Read the model definition and answer for the solid it produces. Units are mm, in the model's axes. Face numbers are marked on the shaded views. A direction names the side the tool comes from. Give positions to 0.01 mm unless a question says otherwise; leave off trailing zeros. Order: outer loops, then holes, each group sorted by start corner. A loop starts at its lowest first (then second) coordinate and runs counter-clockwise, first axis right, second up. Notation, with made-up numbers: M 37,-3.75 L 51,-3.75 A25 ccw 51,10.25 Z; hole C -14.75,59.25 d6. An arc over 180 degrees is marked long. One line per item, written item: value. Start each with the question number.
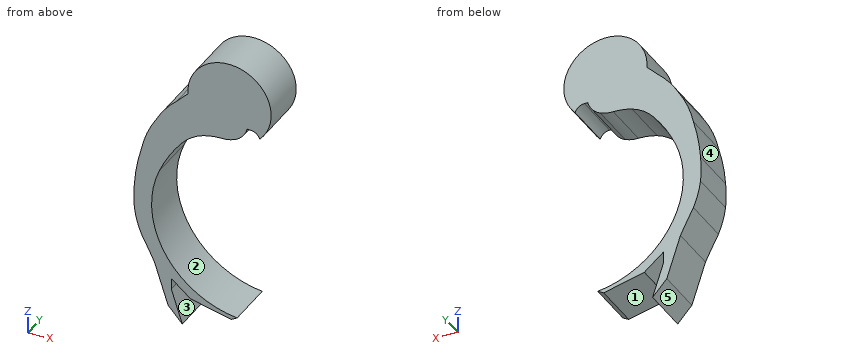
from build123d import *

# Parameters (mm, degrees)
BOSS_EXTRUDE1_DEPTH = 10


with BuildPart() as part:
    # sungu kiri → Boss-Extrude1 (new body)
    with BuildSketch(Plane(origin=(0, 0, 0), x_dir=(1, 0, 0), z_dir=(0, 1, 0))):
        with BuildLine():
            Line((-20.214241335, 18.58200887), (-17.903708636, 25.676772527))
            Line((-17.903708636, 25.676772527), (-20.879327355, 22.419581076))
            Line((-20.879327355, 22.419581076), (-23.726014444, 13.678492013))
            ThreePointArc((-23.726014444, 13.678492013), (-25.061399851, 10.98195956), (-26.444409257, 8.309539974))
            ThreePointArc((-26.444409257, 8.309539974), (-27.383764934, 5.63006722), (-27.936945566, 2.845115782))
            ThreePointArc((-27.936945566, 2.845115782), (-28.068014235, 0.18049064), (-27.936945566, -2.484134502))
            ThreePointArc((-27.936945566, -2.484134502), (-27.425713247, -6.715299694), (-26.444409257, -10.862727794))
            ThreePointArc((-26.444409257, -10.862727794), (-25.296755437, -14.61403578), (-23.488374839, -18.095297119))
            ThreePointArc((-23.488374839, -18.095297119), (-21.509226875, -21.111515913), (-19.028108575, -23.730419207))
            ThreePointArc((-19.028108575, -23.730419207), (-17.889571337, -24.893820319), (-16.718896344, -26.024877014))
            ThreePointArc((-16.718896344, -26.024877014), (-5.074889233, -34.816772241), (-1.682577981, -20.626192702))
            ThreePointArc((-1.682577981, -20.626192702), (-2.440511975, -21.639521262), (-3.645798168, -22.024987085))
            Line((-3.645798168, -22.024987085), (-4.330199558, -22.024987085))
            ThreePointArc((-4.330199558, -22.024987085), (-5.29733591, -20.16091762), (-6.958490383, -18.876132224))
            ThreePointArc((-6.958490383, -18.876132224), (-8.290108773, -18.468617913), (-9.67568618, -18.329152159))
            ThreePointArc((-9.67568618, -18.329152159), (-11.660303974, -18.169286257), (-13.595617391, -17.701496911))
            ThreePointArc((-13.595617391, -17.701496911), (-16.012005666, -16.475638304), (-18.010368345, -14.645827324))
            ThreePointArc((-18.010368345, -14.645827324), (-20.650416196, -11.005311906), (-22.72256926, -7.01414831))
            ThreePointArc((-22.72256926, -7.01414831), (-21.584958488, 10.98418111), (-6.423603233, 20.74980075))
            Line((-6.423603233, 20.74980075), (-7.667855794, 21.470443038))
            Line((-7.667855794, 21.470443038), (-16.17291449, 19.521519125))
            Line((-16.17291449, 19.521519125), (-20.214241335, 16.223172594))
            Line((-20.214241335, 16.223172594), (-20.214241335, 18.58200887))
        make_face()
    extrude(amount=BOSS_EXTRUDE1_DEPTH)


solid = part.part
Q1. A tool of negligible diameter and unlimited length cuts with its end or side. For the marked faces 1 and 2, from which of +Z, -Z, +X, -X, +Y, -Y can it reach the whole face along a straight path? Write none if from no direction.
Q2. Find section A-A, the plane y = 2.25. Give the vertices of the cut face in (x, z).
Q3. Each of these flat-tipped pins is pushed along its axis until it touches: pin 1 (3 mm diameter, centred on y = 2, z = 20, fed in from -X); pin 2 (0.7 mm diameter, centred on y = 3, z = -18, fed in from +X); pin 3 (5 mm diameter, centred on y = 9, z = -16.5, fed in from +X); pin 4 (10 mm diameter, centred on x = -12, z = -19.5, fed in from -Y). Where does it stop, or does it pass through?
Q4. Consider probe 1 along Z at (x, y) = (-9.75, 9.5); probe 2 along Z at (x, y) = (-14.75, 6.5); probe 3 along X at (y, z) = (5.75, -0.5). Determine where each line is inside the solid, lowest interval first.
Q5. Find section B-B, the plane x = -25.25. Give the vertices of the cut face in (y, z), then the cut area to 3 significant figures.
Q6. Determine the mould class of the marked faces 3, 4 and 5 for opening direction Z: released by +Z, released by -Z, zero draft, split by the parting line, or undercut.
Q7. Find section C-C, the plane z = 15.5. Give the vertices of the cut face in (x, y), then the cut area to 3 significant figures.
Evaluation:
1. face 1: -Z, +Y, -Y
1. face 2: +X, +Y, -Y
2. outline: M -27.94,-2.85 A20.14 ccw -26.44,-8.31 A169.62 cw -23.73,-13.68 L -20.88,-22.42 L -17.9,-25.68 L -20.21,-18.58 L -20.21,-16.22 L -16.17,-19.52 L -7.67,-21.47 L -6.42,-20.75 A20 cw -22.72,7.01 A30.3 cw -18.01,14.65 A10 cw -13.6,17.7 A12.71 cw -9.68,18.33 A7.09 ccw -6.96,18.88 A4.88 ccw -4.33,22.02 L -3.65,22.02 A2.08 cw -1.68,20.63 A8.72 ccw long -16.72,26.02 A58.11 ccw -19.03,23.73 A20.33 ccw -23.49,18.1 A21.56 ccw -26.44,10.86 A38.04 ccw -27.94,2.48 A27.15 ccw Z
3. pin 1: x = -23.27
3. pin 2: x = -14.04
3. pin 3: x = -12.76
3. pin 4: y = 0
4. probe 1: -20.99 to -20.11, 18.33 to 35.16
4. probe 2: -19.85 to -17.93, 17.22 to 32.15
4. probe 3: -28.07 to -24.33
5. outline: M 0,-10.61 L 10,-10.61 L 10,14.73 L 0,14.73 Z
5. area: 253 mm2
6. face 3: undercut
6. face 4: released by +Z
6. face 5: released by -Z
7. outline: M -24.91,0 L -17.21,0 L -17.21,10 L -24.91,10 Z
7. area: 77.0 mm2
